from build123d import *

# Parameters (mm, degrees)
EXTRUDE_1_DEPTH           = 127.5
HOLE_WIZARD_1_D           = 3.5
HOLE_WIZARD_1_CBORE_D     = 6.5
HOLE_WIZARD_1_CBORE_DEPTH = 1.8


with BuildPart() as part:
    # 草图1 → 凸台-拉伸1 (new, symmetric)
    with BuildSketch(Plane(origin=(0, 0, 0), x_dir=(0, 0, -1), z_dir=(1, 0, 0))):
        Polygon((-5, -4.35), (-5, -6), (-2.8, -6), (-2.8, 6), (-5, 6), (-5, 4.35), (-6, 4.35), (-6, 7.5), (0, 7.5), (0, -7.5), (-6, -7.5), (-6, -4.35), align=None)
    extrude(amount=EXTRUDE_1_DEPTH, both=True)

    # 孔1 (through all)
    with Locations(Plane.XY.offset(2.8)):
        with Locations((-100, 0), (-50, 0), (0, 0), (50, 0), (100, 0)):
            CounterBoreHole(HOLE_WIZARD_1_D / 2, HOLE_WIZARD_1_CBORE_D / 2, HOLE_WIZARD_1_CBORE_DEPTH)


solid = part.part
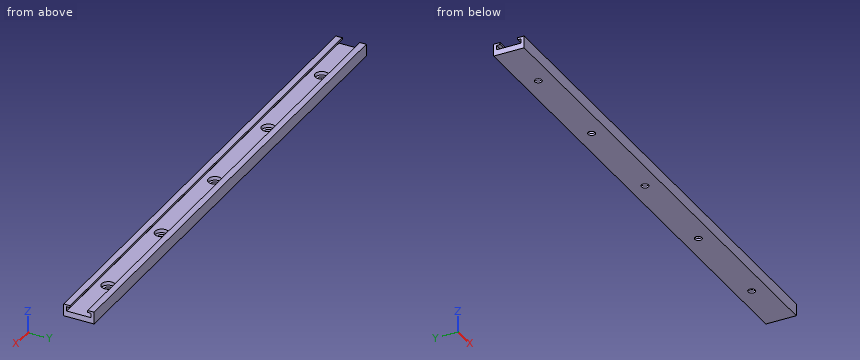
Geometry check sheet. Reference: the model listing, model coordinates, mm. Give positions to 0.01 mm unless a question says otherwise; leave off trailing zeros. Order: outer loops, then holes, each group sorted by start corner. A loop starts at its lowest first (then second) coordinate and runs counter-clockwise, first axis right, second up. Notation, with made-up numbers: (27.25, 38.5) - (59.25, 38.5) arc R21 ccw to (59.25, 46.5) - close; hole circle Ø5 at (9.5, 19.25). An arc over 180 degrees is marked (long way). Answer as a JSON object with one key per item and string values.
(1) Cross-section at A-A (x = 43.5). Record the cut outline in (y, z).
Report:
{"outline": "(-7.5, 0) - (7.5, 0) - (7.5, 6) - (4.35, 6) - (4.35, 5) - (6, 5) - (6, 2.8) - (-6, 2.8) - (-6, 5) - (-4.35, 5) - (-4.35, 6) - (-7.5, 6) - close"}
(2) Depth check by flat-ended pin: pin 1 Ø3 at (x, y) = (19, 4) entering from +Z; pin 2 Ø8.5 at (x, y) = (0, 0) entering from +Z; pin 3 Ø2 at (x, y) = (99.5, -1.5) entering from +Z. Enter the tip coordinate at first touch or a pass-through.
Report:
{"pin 1": "z = 6", "pin 2": "z = 2.8", "pin 3": "z = 1"}
(3) Material ranges on line 1 (Z direction, x = -96.5, y = -5.75); line 2 (X direction, y = 3, z = 2.6); line 3 (Y direction, x = -10, z = 4.5), recorded low to high.
Report:
{"line 1": "0 to 2.8, 5 to 6", "line 2": "-127.5 to -101.25, -98.75 to -51.25, -48.75 to -1.25, 1.25 to 48.75, 51.25 to 98.75, 101.25 to 127.5", "line 3": "-7.5 to -6, 6 to 7.5"}
